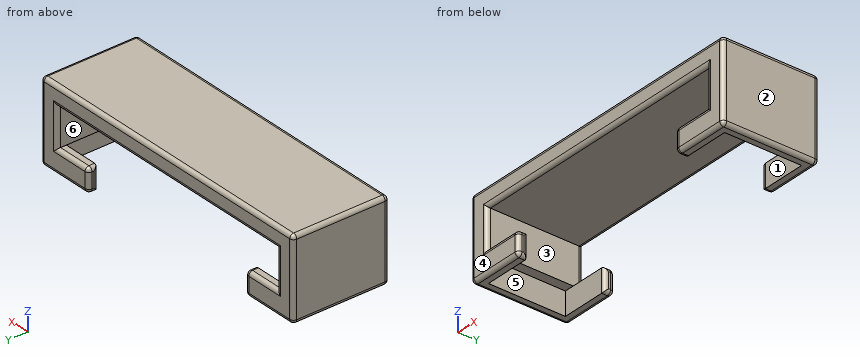
```python
from build123d import *

# Parameters (mm, degrees)
F1_DEPTH    = 25
F2_T        = 2.5
F2_T3_DEPTH = 30
F3_R        = 1


# Not quite as in the source:
# - a shell that OpenCascade refuses in one call is made with other operations: the cavity is built on its own and cut out


with BuildPart() as f1:
    # F0 (on Front) → F1 (new body)
    with BuildSketch(Plane.XZ):
        Polygon((-48.0838582665, 23.83404883), (-48.0838582665, 33.83404883), (21.9161417335, 33.83404883), (21.9161417335, 23.83404883), (11.9161417335, 23.83404883), (11.9161417335, 17.83404883), (21.9161417335, 17.83404883), (26.9161417335, 17.83404883), (26.9161417335, 38.83404883), (-53.0838582665, 38.83404883), (-53.0838582665, 17.83404883), (-48.0838582665, 17.83404883), (-38.0838582665, 17.83404883), (-38.0838582665, 23.83404883), align=None)
    extrude(amount=F1_DEPTH)

    # F2: shell of thickness 2.5, made by hand


with BuildPart() as f2_core1:
    # F2_t2: copy of F1
    add(f1.part)

    # the walls: a layer under each face that stays
    f2_faces = [f2_core1.faces().sort_by_distance(p)[0] for p in [
        (21.9161417335, -12.5, 28.83404883),
        (-39.7505249331, -25, 21.33404883),
        (-48.0838582665, -12.5, 28.83404883),
        (-53.0838582665, -12.5, 28.33404883),
        (-13.0838582665, -12.5, 38.83404883),
        (26.9161417335, -12.5, 28.33404883),
        (-39.7505249331, 0, 21.33404883),
        (-13.0838582665, -12.5, 33.83404883),
    ]]
    thicken(f2_faces, amount=-F2_T, mode=Mode.SUBTRACT)

    # F2_s4 → F2_t3 (cut)
    with BuildSketch(Plane.XZ.offset(-2.5)):
        Polygon((21.8911417335, 33.80904883), (24.4161417335, 33.83404883), (24.4161417335, 36.33404883), (21.9161417335, 36.33404883), align=None)
        Polygon((-48.0588582665, 33.80904883), (-50.5838582665, 33.83404883), (-50.5838582665, 36.33404883), (-48.0838582665, 36.33404883), align=None)
    extrude(amount=F2_T3_DEPTH, mode=Mode.SUBTRACT)


with BuildPart() as f1_1:
    add(f1.part)

    # what is left inside the walls is the cavity
    f2_cavity = [f2_core1.part.solids().sort_by_distance(p)[0] for p in [
        (18.166142, -15.833333, 23.809049),
        (-44.333858, -15.833333, 23.809049),
    ]]
    add(f2_cavity, mode=Mode.SUBTRACT)

    # F3
    f3_edges = [f1_1.edges().sort_by_distance(p)[0] for p in [
        (-38.083858, 0, 20.834049),
        (-38.083858, -1.25, 23.834049),
        (-38.083858, -2.5, 20.834049),
        (-38.083858, -1.25, 17.834049),
        (-38.083858, -22.5, 20.834049),
        (-38.083858, -23.75, 23.834049),
        (-38.083858, -25, 20.834049),
        (-38.083858, -23.75, 17.834049),
        (11.916142, 0, 20.834049),
        (11.916142, -1.25, 17.834049),
        (11.916142, -2.5, 20.834049),
        (11.916142, -1.25, 23.834049),
        (11.916142, -22.5, 20.834049),
        (11.916142, -23.75, 17.834049),
        (11.916142, -25, 20.834049),
        (11.916142, -23.75, 23.834049),
        (21.916142, 0, 28.834049),
        (16.916142, 0, 23.834049),
        (19.416142, 0, 17.834049),
        (26.916142, 0, 28.334049),
        (-13.083858, 0, 38.834049),
        (-53.083858, 0, 28.334049),
        (-45.583858, 0, 17.834049),
        (-43.083858, 0, 23.834049),
        (-48.083858, 0, 28.834049),
        (-13.083858, 0, 33.834049),
        (26.916142, -12.5, 17.834049),
        (26.916142, -12.5, 38.834049),
        (26.916142, -25, 28.334049),
        (21.916142, -25, 28.834049),
        (16.916142, -25, 23.834049),
        (19.416142, -25, 17.834049),
        (-13.083858, -25, 38.834049),
        (-53.083858, -25, 28.334049),
        (-45.583858, -25, 17.834049),
        (-43.083858, -25, 23.834049),
        (-48.083858, -25, 28.834049),
        (-13.083858, -25, 33.834049),
        (-53.083858, -12.5, 38.834049),
        (-53.083858, -12.5, 17.834049),
    ]]
    fillet(f3_edges, radius=F3_R)


solid = f1_1.part
```
Design review of the part built by this model. Coordinates are the model's own, in mm. Face numbers are marked on the shaded views. A direction names the side the tool comes from. Round coordinates to 2 decimals unless told otherwise and drop trailing zeros. Write each loop counter-clockwise with the first axis right and the second up, starting at its lowest first coordinate (ties: lowest second). Pieces come first, ordered by that corner, then holes. Notation, with made-up numbers: (59.25, 44.25) -> (87.25, 44.25) arc R16 cw to (87.25, 63.25) -> close; hole circle Ø3 at (34, -12). An arc over 180 degrees is marked (long way). Answer in a Markdown table with one row per item.
Q1. To check wall thickness, follow L1, parallel to X at y = -11, z = 19; L2, parallel to X at y = -2.25, z = 27.25; L3, parallel to Z at x = -18.5, y = -10.75. State the ranges of each line that lie inside material, in increasing order. Write a range as [from, to].
The answers:
| item | result |
|---|---|
| L1 | [-53.08, -50.58], [24.42, 26.92] |
| L2 | [-53.08, -48.08], [21.92, 26.92] |
| L3 | [33.83, 38.83] |
Q2. Take a section at D-D, the plane y = -11. State the section outline as (x, z) points, then the cut area to 3 significant figures.
The answers:
| item | result |
|---|---|
| outline | (-53.08, 18.83) arc R1 ccw to (-52.08, 17.83) -> (-50.58, 17.83) -> (-50.58, 23.83) -> (-48.08, 23.83) -> (-48.08, 33.83) -> (21.92, 33.83) -> (21.92, 23.83) -> (24.42, 23.83) -> (24.42, 17.83) -> (25.92, 17.83) arc R1 ccw to (26.92, 18.83) -> (26.92, 37.83) arc R1 ccw to (25.92, 38.83) -> (-52.08, 38.83) arc R1 ccw to (-53.08, 37.83) -> close |
| area | 529 mm² |
Q3. Take a section at A-A, the plane z = 19.75. State the section outline as (x, y) points, then the cut area to 3 significant figures.
The answers:
| item | result |
|---|---|
| outline | (-53.08, -24) arc R1 ccw to (-52.08, -25) -> (-39.08, -25) arc R1 ccw to (-38.08, -24) -> (-38.08, -23.5) arc R1 ccw to (-39.08, -22.5) -> (-50.58, -22.5) -> (-50.58, -2.5) -> (-39.08, -2.5) arc R1 ccw to (-38.08, -1.5) -> (-38.08, -1) arc R1 ccw to (-39.08, 0) -> (-52.08, 0) arc R1 ccw to (-53.08, -1) -> close; (11.92, -24) arc R1 ccw to (12.92, -25) -> (25.92, -25) arc R1 ccw to (26.92, -24) -> (26.92, -1) arc R1 ccw to (25.92, 0) -> (12.92, 0) arc R1 ccw to (11.92, -1) -> (11.92, -1.5) arc R1 ccw to (12.92, -2.5) -> (24.42, -2.5) -> (24.42, -22.5) -> (12.92, -22.5) arc R1 ccw to (11.92, -23.5) -> close |
| area | 247 mm² |
Q4. Draft analysis for pull direction Y (two halves, no side actions). For the marked faces 4, 5 and 6, state which applies: +Y half, -Y half, draft (parallel to the pull), parting line (faces both ways), or undercut.
The answers:
| item | result |
|---|---|
| face 4 | -Y half |
| face 5 | undercut |
| face 6 | draft |
Q5. For the marked faces 1, 2 and 3, list the 3-axis set-ups (+Z, -Z, +X, -X, +Y, -Y) from which the entire face can be reached by the end or side of a thin tool; tool diameter is ignored.
The answers:
| item | result |
|---|---|
| face 1 | -Z |
| face 2 | +Z, -Z, +X, +Y, -Y |
| face 3 | +Y, -Y |
Q6. Clearance check with flat-ended pins moving along their axes: pin 1 Ø0.8 at (x, y) = (-49.5, -10.5) entering from -Z; pin 2 Ø5 at (x, y) = (-12.5, -9) entering from -Z. State where each tip first meets the part, or that it passes through.
The answers:
| item | result |
|---|---|
| pin 1 | z = 23.83 |
| pin 2 | z = 33.83 |
Q7. Take a section at C-C, the plane z = 29.5. State the section outline as (x, y) points.
The answers:
| item | result |
|---|---|
| outline | (-53.08, -24) arc R1 ccw to (-52.08, -25) -> (-49.08, -25) arc R1 ccw to (-48.08, -24) -> (-48.08, -1) arc R1 ccw to (-49.08, 0) -> (-52.08, 0) arc R1 ccw to (-53.08, -1) -> close; (21.92, -24) arc R1 ccw to (22.92, -25) -> (25.92, -25) arc R1 ccw to (26.92, -24) -> (26.92, -1) arc R1 ccw to (25.92, 0) -> (22.92, 0) arc R1 ccw to (21.92, -1) -> close |
Q8. Take a section at B-B, the plane x = -43. State the section outline as (y, z) points.
The answers:
| item | result |
|---|---|
| outline | (-25, 18.83) arc R1 ccw to (-24, 17.83) -> (-22.5, 17.83) -> (-22.5, 23.83) -> (-24, 23.83) arc R1 ccw to (-25, 22.83) -> close; (-25, 34.83) arc R1 ccw to (-24, 33.83) -> (-1, 33.83) arc R1 ccw to (0, 34.83) -> (0, 37.83) arc R1 ccw to (-1, 38.83) -> (-24, 38.83) arc R1 ccw to (-25, 37.83) -> close; (-2.5, 17.83) -> (-1, 17.83) arc R1 ccw to (0, 18.83) -> (0, 22.83) arc R1 ccw to (-1, 23.83) -> (-2.5, 23.83) -> close |
